For this review, take the finished solid that the model builds, in its own axes (mm). Give positions to 0.01 mm unless a question says otherwise; leave off trailing zeros. Write each loop counter-clockwise with the first axis right and the second up, starting at its lowest first coordinate (ties: lowest second). Pieces come first, ordered by that corner, then holes.
Q1. We need section A-A (y = -38). Write out the cut boundary in (x, z), then the cut area to 3 significant figures.
Q2. For line 1 (X direction, y = -41.5, z = -27.5); line 2 (Z direction, x = 53.5, y = -45); line 3 (X direction, y = -43, z = -47.25), list the stretches that pass through material, from the lowest coordinate up.
Q3. We need section B-B (z = -28). Write out the cut boundary in (x, y).
```python
from build123d import *

# Parameters (mm, degrees)
F0_W     = 34.1916419566
F0_H     = 22.5922781974
F1_DEPTH = 48.006
F2_SIZE  = 5.08
F3_D     = 5.5


with BuildPart() as f1:
    # F0 (on Front) → F1 (new body)
    with BuildSketch(Plane.XZ):
        with Locations((38.2087547332, -37.4044654891)):
            Rectangle(F0_W, F0_H)
    extrude(amount=F1_DEPTH)

    # F2
    f2_edges = [f1.edges().sort_by_distance(p)[0] for p in [
        (55.304576, -24.003, -48.700605),
    ]]
    chamfer(f2_edges, length=F2_SIZE)

    # F3 (through all)
    with Locations(Plane(origin=(0, 0, 0), x_dir=(1, 0, 0), z_dir=(0, 1, 0))):
        with Locations((55.3045757115, 48.7006045878), (55.3045757115, 26.1083263904), (21.1129337549, 48.7006045878), (21.1129337549, 26.1083263904)):
            Hole(F3_D / 2)


solid = f1.part
```
Computed:
1. outline: (21.11, -45.95) arc R2.75 cw to (23.86, -48.7) - (50.22, -48.7) - (55.3, -43.62) - (55.3, -28.86) arc R2.75 cw to (52.55, -26.11) - (23.86, -26.11) arc R2.75 cw to (21.11, -28.86) - close
1. area: 742 mm2
2. line 1: x = 23.48 to 52.93
2. line 2: z = -45.43 to -28.18
2. line 3: x = 23.45 to 51.68
3. outline: (23.11, -48.01) - (53.31, -48.01) - (53.31, 0) - (23.11, 0) - close
